Can you work these out from the model? Positions are in its coordinate system, mm. A direction names the side the tool comes from. Coordinates: 2 decimals unless noted, no trailing zeros. Order: outer loops, then holes, each group sorted by start corner. A loop starts at its lowest first (then second) coordinate and runs counter-clockwise, first axis right, second up.
```python
from build123d import *

# Parameters (mm, degrees)
SKETCH1_W                    = 55
SKETCH1_H                    = 50
BOSS_EXTRUDE1_DEPTH          = 7
SKETCH6_W                    = 15.2
SKETCH6_H                    = 10
CUT_EXTRUDE1_DEPTH           = 10
M5_CLEARANCE_HOLE1_OUTLINE_R = 2.65
M5_CLEARANCE_HOLE1_DEPTH     = 7
F_4_4_4_4_DIAMETER_HOLE2_D   = 4.4
F_7_8_7_8_DIAMETER_HOLE1_D   = 7.8
FILLET1_R                    = 4
FILLET2_R                    = 1.5
CHAMFER1_SIZE                = 1


# Read off the part's stored shape, not the designer's step: M5 Clearance Hole1
with BuildPart() as part:
    # Sketch1 → Boss-Extrude1 (new body)
    with BuildSketch(Plane(origin=(0, 0, 0), x_dir=(1, 0, 0), z_dir=(0, 1, 0))):
        with Locations((7.5, 25)):
            Rectangle(SKETCH1_W, SKETCH1_H)
    extrude(amount=BOSS_EXTRUDE1_DEPTH)

    # Sketch6 → Cut-Extrude1 (cut)
    with BuildSketch(Plane.XZ):
        with Locations((17.4, -25)):
            Rectangle(SKETCH6_W, SKETCH6_H)
        with BuildLine():
            Line((9.8, -30), (25, -30))
            ThreePointArc((25, -30), (17.4, -37.6), (9.8, -30))
        make_face()
    extrude(amount=-CUT_EXTRUDE1_DEPTH, mode=Mode.SUBTRACT)

    # M5 Clearance Hole1 outline → M5 Clearance Hole1 (cut)
    with BuildSketch(Plane(origin=(0, 0, 0), x_dir=(1, 0, 0), z_dir=(0, 1, 0))):
        with Locations((-10, 10)):
            Circle(M5_CLEARANCE_HOLE1_OUTLINE_R)
        with Locations((27.5, 10)):
            Circle(M5_CLEARANCE_HOLE1_OUTLINE_R)
    extrude(amount=M5_CLEARANCE_HOLE1_DEPTH, mode=Mode.SUBTRACT)

    # Ø4.4 (4.4) Diameter Hole2 (through all)
    with Locations(Plane.XZ):
        with Locations((30, -43), (5, -35), (30, -35), (5, -43)):
            Hole(F_4_4_4_4_DIAMETER_HOLE2_D / 2)

    # Ø7.8 (7.8) Diameter Hole1 (through all)
    with Locations(Plane.XZ):
        with Locations((-10, -35)):
            Hole(F_7_8_7_8_DIAMETER_HOLE1_D / 2)

    # Fillet1
    fillet1_edges = [part.edges().sort_by_distance(p)[0] for p in [
        (35, 3.5, -50),
        (35, 3.5, 0),
        (-20, 3.5, 0),
        (-20, 3.5, -50),
    ]]
    fillet(fillet1_edges, radius=FILLET1_R)

    # Fillet2
    fillet2_edges = [part.edges().sort_by_distance(p)[0] for p in [
        (7.5, 0, 0),
        (7.5, 7, 0),
        (-20, 0, -25),
        (7.5, 0, -50),
        (35, 0, -25),
        (33.828427125, 0, -1.171572875),
        (33.828427125, 0, -48.828427125),
        (-18.828427125, 0, -48.828427125),
        (-18.828427125, 0, -1.171572875),
        (-20, 7, -25),
        (7.5, 7, -50),
        (35, 7, -25),
        (33.828427125, 7, -1.171572875),
        (33.828427125, 7, -48.828427125),
        (-18.828427125, 7, -48.828427125),
        (-18.828427125, 7, -1.171572875),
        (25, 0, -25),
        (17.4, 0, -20),
        (9.8, 0, -25),
        (17.4, 0, -37.6),
    ]]
    fillet(fillet2_edges, radius=FILLET2_R)

    # Chamfer1
    chamfer1_edges = [part.edges().sort_by_distance(p)[0] for p in [
        (-6.1, 0, -35),
    ]]
    chamfer(chamfer1_edges, length=CHAMFER1_SIZE)


solid = part.part
```
1. I'm going to push a flat-ended pin straight in: pin 1 (12.5 mm diameter, centred on x = -10, z = -35, fed in from -Y). Where does the tip first touch, or does it pass through?
Completed:
pin 1: stops at y = 0
2. Imagine slicing it at A-A on x = 17.4. Please give me the cut outline in (y, z), then the cut area to 3 significant figures.
Completed:
outline: (0, -48.5) arc R1.5 ccw to (1.5, -50) - (5.5, -50) arc R1.5 ccw to (7, -48.5) - (7, -37.6) - (1.5, -37.6) arc R1.5 ccw to (0, -39.1) - close; (0, -18.5) arc R1.5 ccw to (1.5, -20) - (7, -20) - (7, -1.5) arc R1.5 ccw to (5.5, 0) - (1.5, 0) arc R1.5 ccw to (0, -1.5) - close
area: 224 mm2
3. Imagine slicing it at C-C on x = 5. Please give me the cut outline in (y, z), then the cut area to 3 significant figures.
Completed:
outline: (0, -48.5) arc R1.5 ccw to (1.5, -50) - (5.5, -50) arc R1.5 ccw to (7, -48.5) - (7, -45.2) - (0, -45.2) - close; (0, -40.8) - (7, -40.8) - (7, -37.2) - (0, -37.2) - close; (0, -32.8) - (7, -32.8) - (7, -1.5) arc R1.5 ccw to (5.5, 0) - (1.5, 0) arc R1.5 ccw to (0, -1.5) - close
area: 286 mm2
4. Thinking about a two-plate mould opening in Z: for faces 4 (the cylindrical face through (7.17, 6.57, -49.55)), 5 (the flat face through (17, 4, -20)), 6 (the cylindrical face through (-19.55, 0.43, -24.71)), which applies, pulls with the +Z half, pulls with the -Z half, needs draft (parallel to the pull), parting line crosses it, or undercut?
Completed:
face 4: pulls with the -Z half
face 5: undercut
face 6: needs draft
5. On a 3-axis mill with a long thin cutter (end or side, diameter ignored), from which of +Z, -Z, +X, -X, +Y, -Y can I reach the whole of each face in a straight line? I mean faces 1 (the cylindrical face through (33.797, 3.528, -1.141)), 2 (the flat face through (25, 4, -25)), 3 (the cylindrical face through (17.53, 0.43, -19.55)). Say none if no direction works.
Completed:
face 1: +Z, +X, +Y, -Y
face 2: +Y, -Y
face 3: -Y
6. Please list where these lines run through material, in increasing order: probe 1 along Z at (x, y) = (-10, 3.4); probe 2 along X at (y, z) = (2, -10); probe 3 along Z at (x, y) = (5, 5.5).
Completed:
probe 1: z = -50 to -38.9, -31.1 to -12.65, -7.35 to 0
probe 2: x = -20 to -12.65, -7.35 to 24.85, 30.15 to 35
probe 3: z = -50 to -45.2, -40.8 to -37.2, -32.8 to 0
7. Imagine slicing it at D-D on z = -12. Please give me the cut outline in (x, y).
Completed:
outline: (-20, 1.5) arc R1.5 ccw to (-18.5, 0) - (-11.74, 0) - (-11.74, 7) - (-18.5, 7) arc R1.5 ccw to (-20, 5.5) - close; (-8.26, 0) - (25.76, 0) - (25.76, 7) - (-8.26, 7) - close; (29.24, 0) - (33.5, 0) arc R1.5 ccw to (35, 1.5) - (35, 5.5) arc R1.5 ccw to (33.5, 7) - (29.24, 7) - close
8. Imagine slicing it at B-B on y = 3. Give the number of separate pieces and of enclosed holes in the cut face, then the cut area to 3 significant figures.
Completed:
separate pieces: 1
enclosed holes: 8
area: 2,340 mm2
